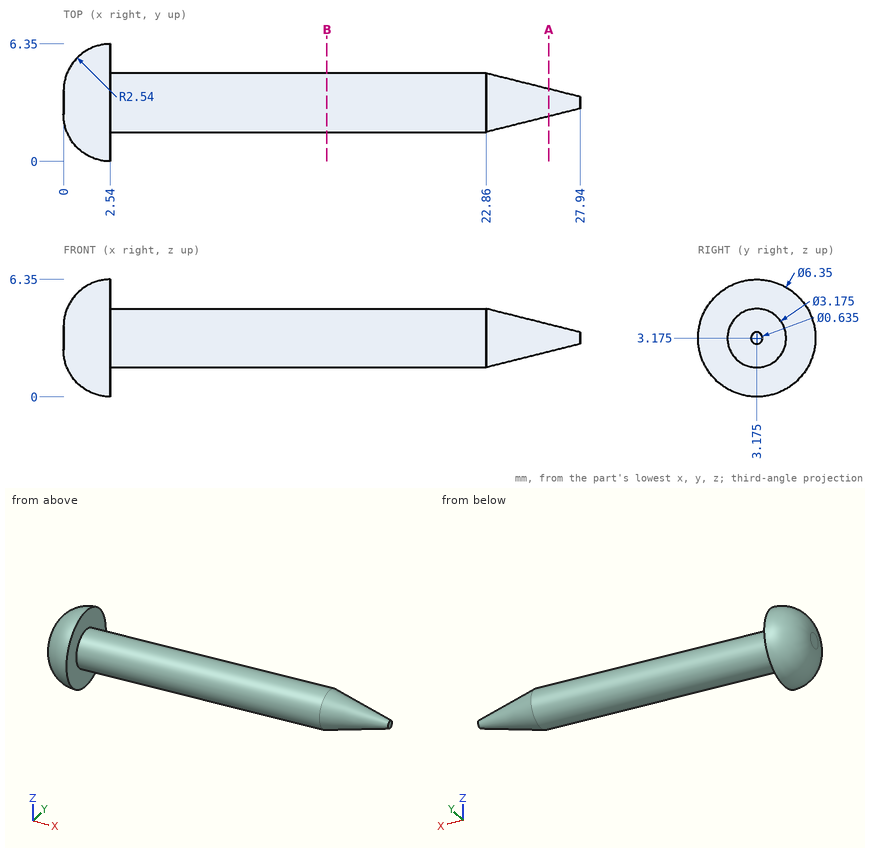
Geometry: see drawing. Coordinates: mm, zero at the bounding-box minimum. Coordinates: 2 decimals unless noted, no trailing zeros. Loops run counter-clockwise (first coordinate to the right, second up) from the corner with the lowest first, then second, coordinate; pieces in that order, holes last. Notation, with made-up numbers: (5, 5.25) - (23, 5.25) arc R21 ccw to (23, 42.25) - close; hole circle Ø9 at (29.25, -22.75). An arc over 180 degrees is marked (long way). Return JSON: item names as keys, results as strings.
Q1. Material intervals for line 1 along Y through (x, z) = (8.25, 4); line 2 along Y through (x, z) = (14.25, 3); line 3 along X through (y, z) = (0.75, 3), sorted ascending.
Results:
{"line 1": "1.82 to 4.53", "line 2": "1.6 to 4.75", "line 3": "0.74 to 2.54"}
Q2. Section B-B, the plane x = 14.25. Return loops of the section in (y, z) (1 decimal), plus the area to 3 significant figures.
Results:
{"outline": "circle Ø3.2 at (3.2, 3.2)", "area": "7.92 mm2"}
Q3. Section A-A, the plane x = 26.25. Return loops of the section in (y, z) (3 decimals).
Results:
{"outline": "circle Ø1.48 at (3.175, 3.175)"}
Q4. Contact query for flat-ended pins moving along their axis: P1, Ø1, axis at x = 9, y = 5, coming from the -Z side; P2, Ø1.5, axis at x = 23, z = 1.5, coming from the -Y side. Output: stop coordinate, or through.
Results:
{"P1": "z = 2.3", "P2": "y = 1.89"}
